```python
from build123d import *

# Parameters (mm, degrees)
F7_W           = 10
F7_H           = 60
F7_W_2         = 40
F0_DEPTH       = 10
F1_DEPTH       = 25
F2_W           = 10
F2_H           = 6
F3_DEPTH       = 15
F6_D           = 8.8
F6_DEPTH       = 25
F6_CSINK_D     = 11
F6_CSINK_ANGLE = 90


with BuildPart() as f0:
    # F7 (on Top) → F0 (new body)
    with BuildSketch(Plane.XY):
        with Locations((-45, 0)):
            Rectangle(F7_W, F7_H)
        Polygon((10, 30), (0, 30), (0, -30), (10, -30), (25, -15), (25, 15), align=None)
        with Locations((-20, 0)):
            Rectangle(F7_W_2, F7_H)
    extrude(amount=F0_DEPTH)

    # F7 (on Top) → F1 (join)
    with BuildSketch(Plane.XY):
        with Locations((-45, 0)):
            Rectangle(F7_W, F7_H)
        Polygon((10, 30), (0, 30), (0, -30), (10, -30), (25, -15), (25, 15), align=None)
    extrude(amount=F1_DEPTH)

    # F2 (on face) → F3 (cut)
    with BuildSketch(Plane.XY.offset(25)):
        with Locations((-45, 0)):
            Rectangle(F2_W, F2_H)
    extrude(amount=-F3_DEPTH, mode=Mode.SUBTRACT)

    # F6
    with Locations(Plane.YZ.offset(25)):
        with Locations((0, 17.5)):
            CounterSinkHole(F6_D / 2, F6_CSINK_D / 2, depth=F6_DEPTH, counter_sink_angle=F6_CSINK_ANGLE)


solid = f0.part
```
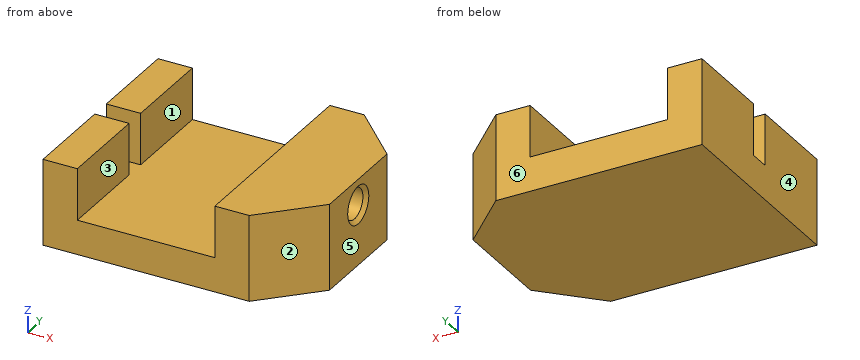
Check sheet for the modelled part. Datum: model origin and axes. Units: mm. Face numbers are marked on the shaded views. A direction names the side the tool comes from. Give positions to 0.01 mm unless a question says otherwise; leave off trailing zeros. Write each loop counter-clockwise with the first axis right and the second up, starting at its lowest first coordinate (ties: lowest second). Pieces come first, ordered by that corner, then holes. Notation, with made-up numbers: (52, -16) -> (93, -16) arc R30 ccw to (93, 7) -> close; hole circle Ø2 at (74, 73.5). An arc over 180 degrees is marked (long way). Use CSV: the item, a comma, the result in double quotes. Start each with the question number.
Q1. Cross-section at D-D on y = 17.5. Enter the section's corners in (x, z), and give its area (3 significant figures).
Q2. Tool access check on the marked faces 1 and 2. Record the directions out of +Z, -Z, +X, -X, +Y, -Y that give a thin tool (end or side, any length) a straight path to the whole face; none if there is none.
Q3. Depth check by flat-ended pin: P1, Ø12, axis at y = -2.5, z = 15.5, coming from the -X side; P2, Ø6, axis at x = -4, y = -4, coming from the +Z side; P3, Ø5.5, axis at y = 0, z = 17.5, coming from the -X side. Enter the tip coordinate at first touch or a pass-through.
Q4. Cross-section at B-B on y = 0. Enter the section's corners in (x, z).
Q5. Release check for a two-part mould opening along X. For the marked faces 3, 4, 5 and 6 record: +X half, -X half, draft (parallel to the pull), parting line (faces both ways), or undercut.
Q6. Cross-section at C-C on x = 14. Enter the section's corners in (y, z).
Q7. Cross-section at A-A on z = 17.5. Enter the section's corners in (x, y), and give its area (3 significant figures).
Q8. Scan lines: line 1 along Y through (x, z) = (6.5, 17.5); line 2 along X through (y, z) = (12.5, 12.5); line 3 along Z through (x, y) = (8, 0). Record each from-to range of solid material in increasing order.
Working result:
1,outline,"(-50, 0) -> (22.5, 0) -> (22.5, 25) -> (0, 25) -> (0, 10) -> (-40, 10) -> (-40, 25) -> (-50, 25) -> close"
1,area,"1,210 mm^2"
2,face 1,"+Z, +Y, -Y"
2,face 2,"+Z, -Z, +X, -Y"
3,P1,"stops at x = -50"
3,P2,"stops at z = 10"
3,P3,"passes through"
4,outline,"(-50, 0) -> (25, 0) -> (25, 12) -> (23.9, 13.1) -> (0, 13.1) -> (0, 10) -> (-50, 10) -> close; (0, 21.9) -> (23.9, 21.9) -> (25, 23) -> (25, 25) -> (0, 25) -> close"
5,face 3,"undercut"
5,face 4,"-X half"
5,face 5,"+X half"
5,face 6,"draft"
6,outline,"(-26, 0) -> (26, 0) -> (26, 25) -> (-26, 25) -> close; hole circle Ø8.8 at (0, 17.5)"
7,outline,"(-50, -30) -> (-40, -30) -> (-40, -3) -> (-50, -3) -> close; (-50, 3) -> (-40, 3) -> (-40, 30) -> (-50, 30) -> close; (0, -30) -> (10, -30) -> (25, -15) -> (25, -5.5) -> (23.9, -4.4) -> (0, -4.4) -> close; (0, 4.4) -> (23.9, 4.4) -> (25, 5.5) -> (25, 15) -> (10, 30) -> (0, 30) -> close"
7,area,"1,590 mm^2"
8,line 1,"y = -30 to -4.4, 4.4 to 30"
8,line 2,"x = -50 to -40, 0 to 25"
8,line 3,"z = 0 to 13.1, 21.9 to 25"
